```python
from build123d import *

# Parameters (mm, degrees)
SALIENTE_EXTRUIR1_DEPTH       = 5
CROQUIS2_R                    = 5
SALIENTE_EXTRUIR2_DEPTH       = 41
CROQUIS3_R                    = 2.5
SALIENTE_EXTRUIR3_DEPTH       = 16
SALIENTE_EXTRUIR10_DEPTH      = 10
SALIENTE_EXTRUIR10_DEPTH_BACK = 7.5
REDONDEO3_R                   = 5
SALIENTE_EXTRUIR11_DEPTH      = 3
CORTAR_EXTRUIR1_DEPTH         = 3


with BuildPart() as part:
    # Croquis1 → Saliente-Extruir1 (new body)
    with BuildSketch(Plane(origin=(0, 0, 0), x_dir=(1, 0, 0), z_dir=(0, 1, 0))):
        Polygon((-50, 15), (-40, 25), (50, 25), (50, -25), (-40, -25), (-50, -15), align=None)
    extrude(amount=SALIENTE_EXTRUIR1_DEPTH)

    # Croquis2 → Saliente-Extruir2 (add, symmetric)
    with BuildSketch(Plane.XY):
        with Locations((-16.666666667, 2.5)):
            Circle(CROQUIS2_R)
    extrude(amount=SALIENTE_EXTRUIR2_DEPTH, both=True)

    # Croquis3 → Saliente-Extruir3 (add)
    with BuildSketch(Plane(origin=(0, 5, 0), x_dir=(1, 0, 0), z_dir=(0, 1, 0))):
        with Locations(Location((0, 0, 0), (0, 0, 270))):
            Circle(CROQUIS3_R)
    extrude(amount=SALIENTE_EXTRUIR3_DEPTH)

    # Croquis24 → Saliente-Extruir10 (add, two sides: drawn at the far end of the back side and taken through both)
    with BuildSketch(Plane.XZ.offset(-SALIENTE_EXTRUIR10_DEPTH_BACK)):
        Polygon((50, 25), (-40, 25), (-50, 15), (-50, -15), (-40, -25), (50, -25), align=None)
        Polygon((46, 22), (-38.757359313, 22), (-47, 13.757359313), (-47, -13.757359313), (-38.757359313, -22), (46, -22), align=None, mode=Mode.SUBTRACT)
    extrude(amount=SALIENTE_EXTRUIR10_DEPTH + SALIENTE_EXTRUIR10_DEPTH_BACK)

    # Redondeo3
    # the kernel refuses this fillet: 5 mm, written as the material it adds along each edge
    with BuildSketch(Plane(origin=(46, 5, -22), x_dir=(0, 0, 1), z_dir=(-1, 0, 0)), Plane(origin=(-23.161857195, 5, 22), x_dir=(0, 0, -1), z_dir=(1, 0, 0))) as redondeo3_piece_1:
        with BuildLine():
            CenterArc((4.330127019, 5), REDONDEO3_R, 210, 60)
            Line((0, 2.5), (0, 0))
            Line((0, 0), (4.330127019, 0))
        make_face()
    extrude(amount=69.161857195)
    with BuildSketch(Plane(origin=(46, 5, 22), x_dir=(-1, 0, 0), z_dir=(0, 0, -1))) as redondeo3_piece_2:
        with BuildLine():
            CenterArc((4.330127019, 5), REDONDEO3_R, 210, 60)
            Line((0, 2.5), (0, 0))
            Line((0, 0), (4.330127019, 0))
        make_face()
    extrude(amount=44)
    with BuildSketch(Plane(origin=(-20.996793686, 5, -22), x_dir=(-1, 0, 0), z_dir=(0, 0, 1))) as redondeo3_piece_3:
        with BuildLine():
            CenterArc((2.284251259, -5), REDONDEO3_R, 90, 41.409622109)
            ThreePointArc((-1.02293788, -1.25), (-0.460660063, -0.66657946), (0, 0))
            Line((0, 0), (2.284251259, 0))
        make_face()
    extrude(amount=44)
    with BuildSketch(Plane(origin=(-12.336539648, 5, -22), x_dir=(-0.6333158920043388, 0.7738933911946454, 0), z_dir=(0, 0, 1))) as redondeo3_piece_4:
        with BuildLine():
            CenterArc((2.422814332, -4.934346413), REDONDEO3_R, 99.295188945, 41.409622109)
            Line((-1.446652623, -1.767766953), (0, 0))
            ThreePointArc((0, 0), (0.807604777, -0.065653587), (1.615209555, 0))
        make_face()
    extrude(amount=44)
    with BuildSketch(Plane(origin=(-49.58267686, 5, 22), x_dir=(0, 0, -1), z_dir=(1, 0, 0))) as redondeo3_piece_5_section:
        with BuildLine():
            CenterArc((4.330127019, 5), REDONDEO3_R, 210, 60)
            Line((0, 2.5), (0, 0))
            Line((0, 0), (4.330127019, 0))
        make_face()
    redondeo3_piece_5 = extrude(amount=39.411200722, mode=Mode.PRIVATE)
    redondeo3_piece_5 = split(redondeo3_piece_5, bisect_by=Plane(origin=(-35.229781416, 5.661212727, 25.527577897), z_dir=(0.7071067811865477, 0, -0.7071067811865475)), keep=Keep.TOP, mode=Mode.PRIVATE)
    add(redondeo3_piece_5)
    with BuildSketch(Plane(origin=(-54.654655446, 5, 6.102703867), x_dir=(0, 1, 0), z_dir=(0.7071067811865475, 0, 0.7071067811865477))) as redondeo3_piece_6_section:
        with BuildLine():
            CenterArc((5, -4.330127019), REDONDEO3_R, 120, 60)
            Line((0, -4.330127019), (0, 0))
            Line((0, 0), (2.5, 0))
        make_face()
    redondeo3_piece_6 = extrude(amount=33.307489344, mode=Mode.PRIVATE)
    redondeo3_piece_6 = split(redondeo3_piece_6, bisect_by=Plane(origin=(-47, 5.661212727, 16.588119965), z_dir=(1, 0, 0)), keep=Keep.TOP, mode=Mode.PRIVATE)
    redondeo3_piece_6 = split(redondeo3_piece_6, bisect_by=Plane(origin=(-41.588119965, 5.661212727, 22), z_dir=(0, 0, -1)), keep=Keep.TOP, mode=Mode.PRIVATE)
    add(redondeo3_piece_6)
    with BuildSketch(Plane(origin=(-47, 5, -24.58267686), x_dir=(1, 0, 0), z_dir=(0, 0, 1))) as redondeo3_piece_7_section:
        with BuildLine():
            CenterArc((4.330127019, 5), REDONDEO3_R, 210, 60)
            Line((0, 2.5), (0, 0))
            Line((0, 0), (4.330127019, 0))
        make_face()
    redondeo3_piece_7 = extrude(amount=49.16535372, mode=Mode.PRIVATE)
    redondeo3_piece_7 = split(redondeo3_piece_7, bisect_by=Plane(origin=(-52.966116147, 5.661212727, 7.791243166), z_dir=(0.7071067811865477, 0, -0.7071067811865475)), keep=Keep.TOP, mode=Mode.PRIVATE)
    redondeo3_piece_7 = split(redondeo3_piece_7, bisect_by=Plane(origin=(-52.966116147, 5.661212727, -7.791243166), z_dir=(0.7071067811865477, 0, 0.7071067811865474)), keep=Keep.TOP, mode=Mode.PRIVATE)
    add(redondeo3_piece_7)
    with BuildSketch(Plane(origin=(-31.102703867, 5, -29.654655446), x_dir=(0.7071067811865478, 0, 0.7071067811865474), z_dir=(-0.7071067811865474, 0, 0.7071067811865477))) as redondeo3_piece_8_section:
        with BuildLine():
            CenterArc((4.330127019, 5), REDONDEO3_R, 210, 60)
            Line((0, 2.5), (0, 0))
            Line((0, 0), (4.330127019, 0))
        make_face()
    redondeo3_piece_8 = extrude(amount=33.307489344, mode=Mode.PRIVATE)
    redondeo3_piece_8 = split(redondeo3_piece_8, bisect_by=Plane(origin=(-47, 5.661212727, -16.588119965), z_dir=(1, 0, 0)), keep=Keep.TOP, mode=Mode.PRIVATE)
    redondeo3_piece_8 = split(redondeo3_piece_8, bisect_by=Plane(origin=(-41.588119965, 5.661212727, -22), z_dir=(0, 0, 1)), keep=Keep.TOP, mode=Mode.PRIVATE)
    add(redondeo3_piece_8)
    with BuildSketch(Plane(origin=(-10.171476138, 5, -22), x_dir=(0, 0, 1), z_dir=(-1, 0, 0))) as redondeo3_piece_9_section:
        with BuildLine():
            CenterArc((4.330127019, 5), REDONDEO3_R, 210, 60)
            Line((0, 2.5), (0, 0))
            Line((0, 0), (4.330127019, 0))
        make_face()
    redondeo3_piece_9 = extrude(amount=39.411200722, mode=Mode.PRIVATE)
    redondeo3_piece_9 = split(redondeo3_piece_9, bisect_by=Plane(origin=(-26.735758427, 5.066113157, -34.021600886), z_dir=(0.7071067811865477, 0, 0.7071067811865474)), keep=Keep.TOP, mode=Mode.PRIVATE)
    add(redondeo3_piece_9)
    with BuildSketch(Plane(origin=(0, 5, 0), x_dir=(0, 0, 1), z_dir=(-1, 0, 0))) as redondeo3_piece_10:
        with BuildLine():
            CenterArc((2.5 + REDONDEO3_R, REDONDEO3_R), REDONDEO3_R, 180, 90)
            Line((2.5, REDONDEO3_R), (2.5, 0))
            Line((2.5, 0), (2.5 + REDONDEO3_R, 0))
        make_face()
    revolve(axis=Axis((0, 5, 0), (0, 1, 0)))

    # Croquis25 → Saliente-Extruir11 (add)
    # profile 1 of 2: a face of its own
    with BuildSketch(Plane.ZY.offset(50)):
        Polygon((-3, 7.5), (-4.271961203, 10.321467355), (-3.825834184, 12.171467355), (-11.478733088, 16.349678992), (-15.514093965, 13.949275268), (-12.566054552, 14.849678992), (-5.713025242, 11.692794832), (-6.047742661, 10.966183347), (-12.344374095, 13.349678992), (-15, 8.75), (-15, 7.5), align=None)
        Polygon((-5.258893064, 11.483596445), (-4.581316792, 11.171467355), (-4.749343557, 10.474693788), (-5.578981907, 10.788740976), align=None, mode=Mode.SUBTRACT)
        with BuildLine():
            Line((-13.556624327, 8.75), (-11.622686259, 12.099678992))
            Line((-11.622686259, 12.099678992), (-4.749343557, 9.974693788))
            Line((-4.749343557, 9.974693788), (-3.915472936, 8.125))
            Line((-3.915472936, 8.125), (-5.723760223, 8.242224542))
            ThreePointArc((-5.723760223, 8.242224542), (-6.834609816, 9.866860567), (-8.145918644, 8.399244067))
            Line((-8.145918644, 8.399244067), (-13.556624327, 8.75))
        make_face(mode=Mode.SUBTRACT)
        with BuildLine():
            ThreePointArc((-6.85573604, 8.822987446), (-7.052684855, 8.457747166), (-6.724418166, 8.711578367))
            add(Edge.make_bspline(
                [(-6.724418166, 8.711578367), (-6.676833807, 8.722274165), (-6.55662927, 8.681929546), (-6.577709986, 8.898272332), (-6.753765056, 8.872588077), (-6.835537659, 8.837673257), (-6.85573604, 8.822987446)],
                knots=[0, 0, 0, 0, 0.159221348, 0.274521525, 0.50339388, 0.587777767, 0.587777767, 0.587777767, 0.587777767], degree=3))
        make_face(mode=Mode.SUBTRACT)
    # profile 2 of 2: a face of its own
    with BuildSketch(Plane.ZY.offset(50)):
        Polygon((15, 7.5), (3, 7.5), (4.271961203, 10.321467355), (3.825834184, 12.171467355), (11.478733088, 16.349678992), (15.514093965, 13.949275268), (12.566054552, 14.849678992), (5.713025242, 11.692794832), (6.047742661, 10.966183347), (12.344374095, 13.349678992), (15, 8.75), align=None)
        Polygon((5.258893064, 11.483596445), (4.581316792, 11.171467355), (4.749343557, 10.474693788), (5.578981907, 10.788740976), align=None, mode=Mode.SUBTRACT)
        with BuildLine():
            Line((3.915472936, 8.125), (5.723760223, 8.242224542))
            ThreePointArc((5.723760223, 8.242224542), (6.834609816, 9.866860567), (8.145918644, 8.399244067))
            Line((8.145918644, 8.399244067), (13.556624327, 8.75))
            Line((13.556624327, 8.75), (11.622686259, 12.099678992))
            Line((11.622686259, 12.099678992), (4.749343557, 9.974693788))
            Line((4.749343557, 9.974693788), (3.915472936, 8.125))
        make_face(mode=Mode.SUBTRACT)
        with BuildLine():
            ThreePointArc((6.85573604, 8.822987446), (7.052684855, 8.457747166), (6.724418166, 8.711578367))
            add(Edge.make_bspline(
                [(6.724418166, 8.711578367), (6.676833807, 8.722274165), (6.55662927, 8.681929546), (6.577709986, 8.898272332), (6.753765056, 8.872588077), (6.835537659, 8.837673257), (6.85573604, 8.822987446)],
                knots=[0, 0, 0, 0, 0.159221348, 0.274521525, 0.50339388, 0.587777767, 0.587777767, 0.587777767, 0.587777767], degree=3))
        make_face(mode=Mode.SUBTRACT)
    extrude(amount=-SALIENTE_EXTRUIR11_DEPTH)

    # Croquis26 → Cortar-Extruir1 (cut)
    with BuildSketch(Plane.ZY.offset(50)):
        Polygon((-6.45713592, -2), (6.45713592, -2), (8.212311407, -0.1), (5.95713592, -0.6), (-5.95713592, -0.6), (-8.212311407, -0.1), align=None)
        Polygon((-0.875, 3.515544457), (0.875, 3.515544457), (0, 2), align=None)
    extrude(amount=-CORTAR_EXTRUIR1_DEPTH, mode=Mode.SUBTRACT)


solid = part.part
```
Here's how the part is built. I have some questions about the finished solid (model axes, mm). A direction names the side the tool comes from. Coordinates: 2 decimals unless noted, no trailing zeros. Loops run counter-clockwise (first coordinate to the right, second up) from the corner with the lowest first, then second, coordinate; pieces in that order, holes last. Notation, with made-up numbers: (-27, -14) - (-8, -14) arc R17 ccw to (-8, 18) - close; hole circle Ø11 at (-12.75, 52.5). An arc over 180 degrees is marked (long way). Return JSON: item names as keys, results as strings. Group by question number.
Item 1: On a 3-axis mill with a long thin cutter (end or side, diameter ignored), from which of +Z, -Z, +X, -X, +Y, -Y can I reach the whole of each face in a straight line? I mean faces 1 (the face through (-41.665, 5.688, 16.549)), 2 (the face through (-48.521, 14.393, -14.061)), 3 (the face through (-21.66, 2.72, 33.11)). Say none if no direction works.
Item 2: If we section it at C-C on x = 15: Write out the boundary of the cut face in (y, z).
Item 3: We'd pull the mould along X, two halves only. Please class faces 4 (the face through (-48.52, 11.05, 8.23)), 5 (the face through (-45.202, 5.688, -0.193)), 6 (the face through (-50, 0, 0)), 7 (the face through (46, -5, 0)): +X half, -X half, draft (parallel to the pull), parting line (faces both ways), or undercut.
Item 4: I need wall thicknesses on line 1 (Z direction, x = 24.5, y = -4.5); line 2 (Y direction, x = 5, z = 18); line 3 (Z direction, x = 7, y = 4). Which ranges of each line are inside material? Lowest first, please. Write a range as from..to.
Item 5: Will these pins go through, and if not, where does the flat tip stop? P1, Ø6, axis at x = -22, z = -10.5, coming from the +Y side; P2, Ø7, axis at y = 13, z = -7, coming from the +X side; P3, Ø8, axis at x = 27, z = -1, coming from the +Y side.
Item 6: If we section it at B-B on x = 0: Write out the boundary of the cut face in (y, z), and give its area (3 significant figures).
Item 7: If we section it at A-A on y = -4.5: Write out the boundary of the cut face in (x, z).
Calculated:
{
 "1": {"face 1": "+Y", "face 2": "+X, -X", "face 3": "+Z"},
 "2": {"outline": "(-10, -25) - (7.5, -25) - (7.5, -22) arc R5 cw to (5, -17.67) - (5, 17.67) arc R5 cw to (7.5, 22) - (7.5, 25) - (-10, 25) - (-10, 22) - (0, 22) - (0, -22) - (-10, -22) - close"},
 "3": {"face 4": "draft", "face 5": "undercut", "face 6": "-X half", "face 7": "undercut"},
 "4": {"line 1": "z = -25..-22, 22..25", "line 2": "y = 0..5.01", "line 3": "z = -25..25"},
 "5": {"P1": "stops at y = 6.92", "P2": "stops at x = -47", "P3": "stops at y = 5"},
 "6": {"outline": "(-10, -25) - (7.5, -25) - (7.5, -22) arc R5 cw to (5, -17.67) - (5, -7.5) arc R5 cw to (10, -2.5) - (21, -2.5) - (21, 2.5) - (10, 2.5) arc R5 cw to (5, 7.5) - (5, 17.67) arc R5 cw to (7.5, 22) - (7.5, 25) - (-10, 25) - (-10, 22) - (0, 22) - (0, -22) - (-10, -22) - close", "area": "422 mm^2"},
 "7": {"outline": "(-50, -15) - (-40, -25) - (50, -25) - (50, 25) - (-40, 25) - (-50, 15) - close; hole (-47, -13.76) - (-38.76, -22) - (46, -22) - (46, 22) - (-38.76, 22) - (-47, 13.76) - close"}
}
